from build123d import *

# Parameters (mm, degrees)
SALIENTE_EXTRUIR1_DEPTH      = 0.8
CROQUIS2_W                   = 36.83
CROQUIS2_H                   = 22.61
SALIENTE_EXTRUIR2_DEPTH      = 3.9
SALIENTE_EXTRUIR2_DEPTH_BACK = 5.1
REDONDEO1_R                  = 1
REDONDEO2_R                  = 1


with BuildPart() as part:
    # Croquis1 → Saliente-Extruir1 (new body)
    with BuildSketch(Plane.XY):
        with BuildLine():
            Line((0, 2), (0, 17.05))
            ThreePointArc((0, 17.05), (0.585786438, 18.464213562), (2, 19.05))
            Line((2, 19.05), (3.62125, 19.05))
            ThreePointArc((3.62125, 19.05), (5.035463562, 18.464213562), (5.62125, 17.05))
            Line((5.62125, 17.05), (5.62125, 9.525))
            ThreePointArc((5.62125, 9.525), (9.59, 5.55625), (13.55875, 9.525))
            Line((13.55875, 9.525), (13.55875, 17.05))
            ThreePointArc((13.55875, 17.05), (14.144536438, 18.464213562), (15.55875, 19.05))
            Line((15.55875, 19.05), (78.91, 19.05))
            ThreePointArc((78.91, 19.05), (80.324213562, 18.464213562), (80.91, 17.05))
            Line((80.91, 17.05), (80.91, 15.49375))
            ThreePointArc((80.91, 15.49375), (80.324213562, 14.079536438), (78.91, 13.49375))
            Line((78.91, 13.49375), (71.31, 13.49375))
            ThreePointArc((71.31, 13.49375), (67.34125, 9.525), (71.31, 5.55625))
            Line((71.31, 5.55625), (78.91, 5.55625))
            ThreePointArc((78.91, 5.55625), (80.324213562, 4.970463562), (80.91, 3.55625))
            Line((80.91, 3.55625), (80.91, 2))
            ThreePointArc((80.91, 2), (80.324213562, 0.585786438), (78.91, 0))
            Line((78.91, 0), (2, 0))
            ThreePointArc((2, 0), (0.585786438, 0.585786438), (0, 2))
        make_face()
    extrude(amount=SALIENTE_EXTRUIR1_DEPTH)

    # Croquis2 → Saliente-Extruir2 (add, two sides)
    with BuildSketch(Plane.XY.offset(0.8)) as saliente_extruir2_sk:
        with Locations((40.455, 9.525)):
            Rectangle(CROQUIS2_W, CROQUIS2_H)
    extrude(amount=SALIENTE_EXTRUIR2_DEPTH)
    extrude(saliente_extruir2_sk.sketch, amount=-SALIENTE_EXTRUIR2_DEPTH_BACK)

    # Redondeo1
    redondeo1_edges = [part.edges().sort_by_distance(p)[0] for p in [
        (22.04, 9.525, -4.3),
        (58.87, 9.525, -4.3),
        (40.455, 20.83, -4.3),
        (40.455, -1.78, -4.3),
    ]]
    fillet(redondeo1_edges, radius=REDONDEO1_R)

    # Redondeo2
    redondeo2_edges = [part.edges().sort_by_distance(p)[0] for p in [
        (22.04, 9.525, 4.7),
        (40.455, -1.78, 4.7),
        (58.87, 9.525, 4.7),
        (40.455, 20.83, 4.7),
    ]]
    fillet(redondeo2_edges, radius=REDONDEO2_R)


solid = part.part
Verification items for the finished model (mm, model axes). A direction names the side the tool comes from. Round coordinates to 2 decimals unless told otherwise and drop trailing zeros. Loops run counter-clockwise (first coordinate to the right, second up) from the corner with the lowest first, then second, coordinate; pieces in that order, holes last. Notation, with made-up numbers: (28.5, 2) - (41.5, 2) arc R16 cw to (41.5, 9) - close; hole circle Ø2 at (18, -12). An arc over 180 degrees is marked (long way). Use one line per item in the form item = value.
1. Scan lines: probe 1 along Y at (x, z) = (74, 0.25); probe 2 along Z at (x, y) = (65, 8.25); probe 3 along X at (y, z) = (16.25, -3.25). Record each from-to range of solid material in increasing order.
A:
probe_1 = 0 to 5.56, 13.49 to 19.05
probe_2 = 0 to 0.8
probe_3 = 22.04 to 58.87
2. Section check B-B on x = 9.59. Record the cut outline in (y, z).
A:
outline = (0, 0) - (5.56, 0) - (5.56, 0.8) - (0, 0.8) - close
3. Section check C-C on z = -1.5. Record the cut outline in (x, y).
A:
outline = (22.04, -1.78) - (58.87, -1.78) - (58.87, 20.83) - (22.04, 20.83) - close
4. Draft check along Y on faces 1 (the flat face through (68, 12, 0)), 2 (the cylindrical face through (0.6, 0.57, 0.39)), 3 (the cylindrical face through (80.34, 14.095, 0.394)). Enter one of: pulls with the +Y half, pulls with the -Y half, needs draft (parallel to the pull), parting line crosses it, or undercut.
A:
face_1 = needs draft
face_2 = pulls with the -Y half
face_3 = undercut
5. Section check A-A on x = 75. Record the cut outline in (y, z).
A:
outline = (0, 0) - (5.56, 0) - (5.56, 0.8) - (0, 0.8) - close; (13.49, 0) - (19.05, 0) - (19.05, 0.8) - (13.49, 0.8) - close
6. Gauge pin test, flat ends, axial feed: pin 1 Ø5 at (x, y) = (22.5, 5) entering from -Z; pin 2 Ø6 at (x, y) = (62, 11.5) entering from +Z; pin 3 Ø0.6 at (x, z) = (3, 0.5) entering from +Y; pin 4 Ø0.6 at (y, z) = (13.5, 0.5) entering from +X. Record the tip position at first contact, or that the pin passes through.
A:
pin_1 = -4.3
pin_2 = 0.8
pin_3 = 19.05
pin_4 = 79.97
7. Access from +Z, -Z, +X, -X, +Y, -Y to the whole of each face (thin tool, end or side, straight path). Record for faces 4 (the cylindrical face through (14.13, 18.45, 0.39)), 5 (the cylindrical face through (80.309, 4.986, 0.394)), 6 (the flat face through (14, 8, 0)), 7 (the flat face through (68, 12, 0.8)).
A:
face_4 = +Z, -Z, +Y
face_5 = +Z, -Z, +X
face_6 = -Z, -X, +Y, -Y
face_7 = +Z, +X, +Y, -Y
